```python
from build123d import *

# Parameters (mm, degrees)
SKETCH1_R           = 1.4
BOSS_EXTRUDE1_DEPTH = 0.8


with BuildPart() as part:
    # Sketch1 → Boss-Extrude1 (new, symmetric)
    with BuildSketch(Plane(origin=(0, 0, 0), x_dir=(0, 0, -1), z_dir=(1, 0, 0))):
        with BuildLine():
            Line((-34.468542217, -41.323283133), (34.440131171, -41.323283133))
            ThreePointArc((34.440131171, -41.323283133), (37.975665077, -39.858817038), (39.440131171, -36.323283133))
            Line((39.440131171, -36.323283133), (39.440131171, 36.293536969))
            ThreePointArc((39.440131171, 36.293536969), (37.975665077, 39.829070875), (34.440131171, 41.293536969))
            Line((34.440131171, 41.293536969), (-28.468542217, 41.293536969))
            Line((-28.468542217, 41.293536969), (-28.468542217, 34.063536969))
            ThreePointArc((-28.468542217, 34.063536969), (-29.200775264, 32.295770016), (-30.968542217, 31.563536969))
            Line((-30.968542217, 31.563536969), (-39.468542217, 31.563536969))
            Line((-39.468542217, 31.563536969), (-39.468542217, -36.323283133))
            ThreePointArc((-39.468542217, -36.323283133), (-38.004076123, -39.858817038), (-34.468542217, -41.323283133))
        make_face()
        with Locations((-35.968542217, 27.793536969)):
            Circle(SKETCH1_R, mode=Mode.SUBTRACT)
        with Locations((22.031457783, 27.493536969)):
            Circle(SKETCH1_R, mode=Mode.SUBTRACT)
        with Locations((-34.468542217, -34.206463031)):
            Circle(SKETCH1_R, mode=Mode.SUBTRACT)
        with Locations((36.031457783, -34.206463031)):
            Circle(SKETCH1_R, mode=Mode.SUBTRACT)
    extrude(amount=BOSS_EXTRUDE1_DEPTH, both=True)


solid = part.part
```
Design review of the part built by this model. Coordinates are the model's own, in mm. Coordinates: 2 decimals unless noted, no trailing zeros. Write each loop counter-clockwise with the first axis right and the second up, starting at its lowest first coordinate (ties: lowest second). Pieces come first, ordered by that corner, then holes. Notation, with made-up numbers: M -35,-36 L 18,-36 A27 ccw 18,-4 Z; hole C 14,57.5 d11. An arc over 180 degrees is marked long. Answer as a JSON object with one key per item and string values.
Item 1: Add section B-B, the plane z = 29.5. Give the boundary of the cut face in (x, y).
Outcome:
{"outline": "M -0.8,-41.32 L 0.8,-41.32 L 0.8,32.04 L -0.8,32.04 Z"}
Item 2: Add section A-A, the plane x = 0.05. Give the boundary of the cut face in (y, z), and give its area (3 significant figures).
Outcome:
{"outline": "M -41.32,-34.44 A5 ccw -36.32,-39.44 L 36.29,-39.44 A5 ccw 41.29,-34.44 L 41.29,28.47 L 34.06,28.47 A2.5 cw 31.56,30.97 L 31.56,39.47 L -36.32,39.47 A5 ccw -41.32,34.47 Z; hole C -34.21,-36.03 d2.8; hole C -34.21,34.47 d2.8; hole C 27.49,-22.03 d2.8; hole C 27.79,35.97 d2.8", "area": "6,370 mm²"}
Item 3: Insertion check: pin 1 Ø2.5 at (y, z) = (-34.21, -36.03) entering from -X. The pin has a flat end and moves straight along its axis. Give the tip position at first contact, or say it passes through.
Outcome:
{"pin 1": "through"}
Item 4: Draft analysis for pull direction Z (two halves, no side actions). For faces 1 (the cylindrical face through (0.011, 32.315, 29.181)), 2 (the flat face through (0.8, 1, 1)), 3 (the cylindrical face through (-0.011, -34.145, 35.867)), state which applies: pulls with the +Z half, pulls with the -Z half, needs draft (parallel to the pull), parting line crosses it, or undercut.
Outcome:
{"face 1": "pulls with the +Z half", "face 2": "needs draft", "face 3": "undercut"}
Item 5: Wall thickness on probe 1 along Y at (x, z) = (0.75, 35); probe 2 along Y at (x, z) = (-0.2, 33.5); probe 3 along Z at (x, y) = (0.6, 36.5): over which ranges is each line inside the solid? List them lowest first.
Outcome:
{"probe 1": "-41.29 to -35.5, -32.91 to 26.78, 28.8 to 31.56", "probe 2": "-41.32 to -35.22, -33.2 to 31.56", "probe 3": "-39.44 to 28.47"}
